```python
from build123d import *

# Parameters (mm, degrees)
BOSS_EXTRU_1_DEPTH = 4
CONG_1_R           = 10


with BuildPart() as part:
    # Esquisse1 → Boss.-Extru.1 (new body)
    with BuildSketch(Plane(origin=(0, 0, 0), x_dir=(0, 0, -1), z_dir=(1, 0, 0))):
        with BuildLine():
            Line((-27.5, 13.15), (-27.5, 0))
            add(Edge.make_bspline(
                [(-27.5, 0), (-6.736181912, -17.460350191), (-2.1, -43)],
                knots=[0, 0, 0, 1, 1, 1], degree=2))
            Line((-2.1, -43), (-2.1, -15))
            Line((-2.1, -15), (2.1, -15))
            Line((2.1, -15), (2.1, -43))
            add(Edge.make_bspline(
                [(27.5, 0), (6.736181912, -17.460350191), (2.1, -43)],
                knots=[0, 0, 0, 1, 1, 1], degree=2))
            Line((27.5, 0), (27.5, 13.15))
            Line((27.5, 13.15), (5.9, 13.15))
            Line((5.9, 13.15), (5.9, 0))
            Line((5.9, 0), (-5.9, 0))
            Line((-5.9, 0), (-5.9, 13.15))
            Line((-5.9, 13.15), (-27.5, 13.15))
        make_face()
    extrude(amount=BOSS_EXTRU_1_DEPTH)

    # Congé1
    cong_1_edges = [part.edges().sort_by_distance(p)[0] for p in [
        (2, 0, -27.5),
        (2, 0, 27.5),
    ]]
    fillet(cong_1_edges, radius=CONG_1_R)


solid = part.part
```
Build history of the part. All positions in model axes, mm. A direction names the side the tool comes from. Round coordinates to 2 decimals unless told otherwise and drop trailing zeros. Answer as CSV lines item,"result".
1. 3-axis set-ups, long thin cutter, end or side, ignore diameter. For faces 1 (the flat face through (2, 7, -5.9)), 2 (the flat face through (2, 13.15, -17)), 3 (the flat face through (2, -29, 2.1)): which of +Z, -Z, +X, -X, +Y, -Y reach the whole face in a straight line?
Resolved:
face 1,"+X, -X, +Y"
face 2,"+Z, -Z, +X, -X, +Y"
face 3,"+X, -X, -Y"
2. Two-plate mould, pull along Z, no slides. Class faces 4 (the flat face through (2, 13.15, 17)), 5 (the flat face through (2, 9, -27.5)), 6 (the flat face through (2, 6, 5.9)): released by +Z, released by -Z, zero draft, split by the parting line, or undercut.
Resolved:
face 4,"zero draft"
face 5,"released by -Z"
face 6,"undercut"
3. Flat gauge pins, fed straight in: P1, Ø1.2, axis at x = 2, y = -34, coming from the -Z side; P2, Ø2, axis at x = 1.5, y = -30, coming from the +Z side; P3, Ø1.2, axis at x = 1.5, z = -2, coming from the +Y side. Where does each tip first touch, or does it go through?
Resolved:
P1,"stops at z = -4.5"
P2,"stops at z = 6.09"
P3,"stops at y = 0"
4. Wall check: probe 1 along Z at (x, y) = (0.85, 8); probe 2 along Y at (x, z) = (1.15, -25); probe 3 along Z at (x, y) = (3.6, -21.5). Give the ranges that are in metal, low to high. Write a range as [from, to].
Resolved:
probe 1,"z = [-27.5, -5.9], [5.9, 27.5]"
probe 2,"y = [-2.11, 13.15]"
probe 3,"z = [-9.62, -2.1], [2.1, 9.62]"
